Read the model definition and answer for the solid it produces. Units are mm, in the model's axes. A direction names the side the tool comes from. Round coordinates to 2 decimals unless told otherwise and drop trailing zeros. Order: outer loops, then holes, each group sorted by start corner. A loop starts at its lowest first (then second) coordinate and runs counter-clockwise, first axis right, second up. Notation, with made-up numbers: (70.5, 54) -> (96.5, 54) arc R31 cw to (96.5, 80) -> close; hole circle Ø3 at (25.25, 62). An arc over 180 degrees is marked (long way). One line per item, written item: value. Start each with the question number.
1. Section A-A (y = -19.5) is taken. Give the vertices of the cut face in (x, z), then the cut area to 3 significant figures.
2. The mould has two halves that part along X. Classify faces 5 (the face through (24, -15.5, 8)), 6 (the face through (-5.1, -4, 4)), 7 (the face through (-26.5, -17, 5)): released by +X, released by -X, zero draft, split by the parting line, or undercut.
3. Consider line 1 (Y direction, x = 0, z = 1.4); line 2 (X direction, y = -23.5, z = 7); line 3 (Z direction, x = 15, y = -3.25). Determine where each line is inside the solid, lowest interval first.
4. Section C-C (z = 9.5) is taken. Give the vertices of the cut face in (x, y).
5. For faces 1 (the face through (-21.5, -20, 5)), 2 (the face through (5.1, -4, 4)), 3 (the face through (0, -8, 6)), 4 (the face through (23, -4, 3)), determine the directions among +Z, -Z, +X, -X, +Y, -Y from which every point of the face is accessible in a straight line to the end or side of a thin tool.
6. Section B-B (x = 0) is taken. Give the vertices of the cut face in (y, z).
7. Flat-ended cylindrical pins translate along their axes: pin 1 Ø5 at (x, y) = (0, -3.5) entering from +Z; pin 2 Ø1.5 at (x, z) = (-0.5, 3) entering from +Y; pin 3 Ø15 at (x, y) = (-5.5, -4) entering from +Z. Find the tip coordinate at first contact, or state that the pin passes through.
8. Section D-D (z = 2.5) is taken. Give the vertices of the cut face in (x, y).
from build123d import *

# Parameters (mm, degrees)
BOSS_EXTRUDE1_DEPTH  = 6
SKETCH6_W            = 5
SKETCH6_H            = 10
BOSS_EXTRUDE2_DEPTH  = 4
SKETCH3_W            = 5.1
SKETCH3_H            = 7.5
CUT_EXTRUDE1_DEPTH   = 4
M4_CLEARANCE_HOLE1_D = 4.5
CHAMFER2_SIZE        = 4


with BuildPart() as part:
    # Sketch1 → Boss-Extrude1 (new body)
    with BuildSketch(Plane.XY):
        Polygon((0, 0), (0, -10), (-19, -10), (-21.5, -12.5), (-21.5, -27.5), (-26.5, -27.5), (-26.5, -7.5), (-19, 0), align=None)
    boss_extrude1 = extrude(amount=BOSS_EXTRUDE1_DEPTH)

    # Sketch6 → Boss-Extrude2 (add)
    with BuildSketch(Plane.XY.offset(6)):
        with Locations((-24, -22.5)):
            Rectangle(SKETCH6_W, SKETCH6_H)
    boss_extrude2 = extrude(amount=BOSS_EXTRUDE2_DEPTH)

    # Sketch3 → Cut-Extrude1 (cut)
    with BuildSketch(Plane.XY.offset(6)):
        with Locations((-2.55, -3.75)):
            Rectangle(SKETCH3_W, SKETCH3_H)
    cut_extrude1 = extrude(amount=-CUT_EXTRUDE1_DEPTH, mode=Mode.SUBTRACT)

    # Mirror1: Boss-Extrude1, Boss-Extrude2, Cut-Extrude1 across plane
    add(boss_extrude1.mirror(Plane(origin=(0, 0, 6), x_dir=(0, 0, 1), z_dir=(-1, 0, 0))))
    add(boss_extrude2.mirror(Plane(origin=(0, 0, 6), x_dir=(0, 0, 1), z_dir=(-1, 0, 0))))
    add(cut_extrude1.mirror(Plane(origin=(0, 0, 6), x_dir=(0, 0, 1), z_dir=(-1, 0, 0))), mode=Mode.SUBTRACT)

    # M4 Clearance Hole1 (through all)
    with Locations(Plane.XY.offset(2)):
        with Locations((0, -3.5)):
            Hole(M4_CLEARANCE_HOLE1_D / 2)

    # Chamfer2
    # the kernel refuses this chamfer: 4 mm, written as the material it adds along each edge
    with BuildSketch(Plane(origin=(-21.5, -17.5, 6), x_dir=(0, 0.9996219169112968, -0.02749587661058627), z_dir=(-1, 0, 0))) as chamfer2_piece_1_section:
        Polygon((CHAMFER2_SIZE * 0.999621916911, -CHAMFER2_SIZE * 0.0274958766106), (-CHAMFER2_SIZE * 0.0274958766106, -CHAMFER2_SIZE * 0.999621916911), (0, 0), align=None)
    chamfer2_piece_1 = extrude(amount=5, mode=Mode.PRIVATE)
    chamfer2_piece_1 = split(chamfer2_piece_1, bisect_by=Plane(origin=(-24, -16.178383383, 10), z_dir=(0, 0, -1)), keep=Keep.TOP, mode=Mode.PRIVATE)
    add(chamfer2_piece_1)
    with BuildSketch(Plane(origin=(21.5, -17.5, 6), x_dir=(0, 0.9996219169112968, -0.02749587661058627), z_dir=(1, 0, 0))) as chamfer2_piece_2_section:
        Polygon((CHAMFER2_SIZE * 0.999621916911, CHAMFER2_SIZE * 0.0274958766106), (-CHAMFER2_SIZE * 0.0274958766106, CHAMFER2_SIZE * 0.999621916911), (0, 0), align=None)
    chamfer2_piece_2 = extrude(amount=5, mode=Mode.PRIVATE)
    chamfer2_piece_2 = split(chamfer2_piece_2, bisect_by=Plane(origin=(24, -16.178383383, 10), z_dir=(0, 0, -1)), keep=Keep.TOP, mode=Mode.PRIVATE)
    add(chamfer2_piece_2)


solid = part.part
Answer:
1. outline: (-26.5, 0) -> (-21.5, 0) -> (-21.5, 10) -> (-26.5, 10) -> close; (21.5, 0) -> (26.5, 0) -> (26.5, 10) -> (21.5, 10) -> close
1. area: 100 mm^2
2. face 5: zero draft
2. face 6: undercut
2. face 7: released by -X
3. line 1: -10 to -5.75, -1.25 to 0
3. line 2: -26.5 to -21.5, 21.5 to 26.5
3. line 3: 0 to 6
4. outline: (-26.5, -27.5) -> (-21.5, -27.5) -> (-21.5, -17) -> (-26.5, -17) -> close; (21.5, -27.5) -> (26.5, -27.5) -> (26.5, -17) -> (21.5, -17) -> close
5. face 1: +Z, -Z, -Y
5. face 2: +Z, +Y
5. face 3: +Z, +X, -X, +Y
5. face 4: +Z, -Z, +X, +Y
6. outline: (-10, 0) -> (-5.75, 0) -> (-5.75, 2) -> (-7.5, 2) -> (-7.5, 6) -> (-10, 6) -> close; (-1.25, 0) -> (0, 0) -> (0, 2) -> (-1.25, 2) -> close
7. pin 1: z = 2
7. pin 2: y = -7.5
7. pin 3: z = 6
8. outline: (-26.5, -27.5) -> (-21.5, -27.5) -> (-21.5, -12.5) -> (-19, -10) -> (19, -10) -> (21.5, -12.5) -> (21.5, -27.5) -> (26.5, -27.5) -> (26.5, -7.5) -> (19, 0) -> (5.1, 0) -> (5.1, -7.5) -> (-5.1, -7.5) -> (-5.1, 0) -> (-19, 0) -> (-26.5, -7.5) -> close
